The listing builds one solid part. Answer for the finished solid, in the listing's coordinates (mm). Coordinates: 2 decimals unless noted, no trailing zeros. Order: outer loops, then holes, each group sorted by start corner. A loop starts at its lowest first (then second) coordinate and runs counter-clockwise, first axis right, second up. Notation, with made-up numbers: (13, -13) -> (57, -13) arc R24 ccw to (57, 2) -> close; hole circle Ø5 at (-10, 57). An arc over 180 degrees is marked (long way). One line per question, with ' | ' between items.
from build123d import *

# Parameters (mm, degrees)
CROQUIS1_R                   = 150
SALIENTE_EXTRUIR1_DEPTH      = 3
REDONDEO1_R                  = 10
TALADRO_DE_MARGEN_PARA_M31_D = 3.4


with BuildPart() as part:
    # Croquis1 → Saliente-Extruir1 (new body)
    with BuildSketch(Plane.XY):
        Circle(CROQUIS1_R)
        with BuildLine():
            Line((9.972316505, -129.616946822), (19.597749078, -19.597749078))
            Line((19.597749078, -19.597749078), (129.616946822, -9.972316505))
            ThreePointArc((129.616946822, -9.972316505), (91.923881554, -91.923881554), (9.972316505, -129.616946822))
        make_face(mode=Mode.SUBTRACT)
        with BuildLine():
            Line((129.616946822, 9.972316505), (15, 20))
            ThreePointArc((15, 20), (0, 25), (-15, 20))
            Line((-15, 20), (-129.616946822, 9.972316505))
            ThreePointArc((-129.616946822, 9.972316505), (0, 130), (129.616946822, 9.972316505))
        make_face(mode=Mode.SUBTRACT)
        with BuildLine():
            Line((-129.616946822, -9.972316505), (-19.597749078, -19.597749078))
            Line((-19.597749078, -19.597749078), (-9.972316505, -129.616946822))
            ThreePointArc((-9.972316505, -129.616946822), (-91.923881554, -91.923881554), (-129.616946822, -9.972316505))
        make_face(mode=Mode.SUBTRACT)
    extrude(amount=SALIENTE_EXTRUIR1_DEPTH)

    # Redondeo1
    redondeo1_edges = [part.edges().sort_by_distance(p)[0] for p in [
        (-129.616946822, 9.972316505, 1.5),
        (-15, 20, 1.5),
        (15, 20, 1.5),
        (129.616946822, 9.972316505, 1.5),
        (9.972316505, -129.616946822, 1.5),
        (129.616946822, -9.972316505, 1.5),
        (19.597749078, -19.597749078, 1.5),
        (-129.616946822, -9.972316505, 1.5),
        (-9.972316505, -129.616946822, 1.5),
        (-19.597749078, -19.597749078, 1.5),
    ]]
    fillet(redondeo1_edges, radius=REDONDEO1_R)

    # Taladro de margen para M31 (through all)
    with Locations(Plane.XY.offset(3)):
        with Locations((0, 10.5), (10.5, 0), (0, -10.5), (-10.5, 0)):
            Hole(TALADRO_DE_MARGEN_PARA_M31_D / 2)


solid = part.part
Item 1: Section C-C, the plane y = -45 is taken. Give the vertices of the cut face in (x, z).
Computed values:
outline: (-143.09, 0) -> (-121.96, 0) -> (-121.96, 3) -> (-143.09, 3) -> close; (-17.38, 0) -> (17.38, 0) -> (17.38, 3) -> (-17.38, 3) -> close; (121.96, 0) -> (143.09, 0) -> (143.09, 3) -> (121.96, 3) -> close
Item 2: Find the intervals of material crossed by L1, parallel to Y at x = -10, z = 0.35; L2, parallel to X at y = -95.5, z = 1.45; L3, parallel to X at y = -60, z = 2.25, in increasing order.
Computed values:
L1: y = -149.67 to -1.62, 1.62 to 22.91, 129.61 to 149.67 | L2: x = -115.67 to -88.2, -12.96 to 12.96, 88.2 to 115.67 | L3: x = -137.48 to -115.33, -16.06 to 16.06, 115.33 to 137.48
Item 3: Determine the mould class of faces 1 (the face through (-19.527, 148.724, 1.479)), 2 (the face through (-2, 2, 3)), 3 (the face through (21.827, -21.689, 1.521)) for opening direction Y: pulls with the +Y half, pulls with the -Y half, needs draft (parallel to the pull), parting line crosses it, or undercut.
Computed values:
face 1: parting line crosses it | face 2: needs draft | face 3: undercut
Item 4: Section B-B, the plane x = -35 is taken. Give the vertices of the cut face in (y, z).
Computed values:
outline: (-145.86, 0) -> (-125.2, 0) -> (-125.2, 3) -> (-145.86, 3) -> close; (-18.25, 0) -> (18.25, 0) -> (18.25, 3) -> (-18.25, 3) -> close; (125.2, 0) -> (145.86, 0) -> (145.86, 3) -> (125.2, 3) -> close
Item 5: This flat-tipped pin is pushed along its axis until it touches: pin 1 Ø2 at (x, y) = (118.5, 46.5) entering from -Z. Where does it stop, or does it pass through?
Computed values:
pin 1: passes through
Item 6: Section A-A, the plane z = 0.8 is taken. Give the vertices of the cut face in (x, y), plus the area to 3 significant figures.
Computed values:
outline: circle Ø300 at (0, 0); hole (-127.99, -22.77) arc R130 ccw to (-22.77, -127.99) arc R10 ccw to (-11.05, -117.27) -> (-18.87, -27.96) arc R10 ccw to (-27.96, -18.87) -> (-117.27, -11.05) arc R10 ccw to start; hole (-127.99, 22.77) arc R10 ccw to (-117.27, 11.05) -> (-17.59, 19.77) arc R10 ccw to (-13.19, 21.24) arc R25 cw to (13.19, 21.24) arc R10 ccw to (17.59, 19.77) -> (117.27, 11.05) arc R10 ccw to (127.99, 22.77) arc R130 ccw to start; hole circle Ø3.4 at (-10.5, 0); hole circle Ø3.4 at (0, -10.5); hole circle Ø3.4 at (0, 10.5); hole circle Ø3.4 at (10.5, 0); hole (11.05, -117.27) arc R10 ccw to (22.77, -127.99) arc R130 ccw to (127.99, -22.77) arc R10 ccw to (117.27, -11.05) -> (27.96, -18.87) arc R10 ccw to (18.87, -27.96) -> close | area: 29,200 mm^2
